```python
from build123d import *

# Parameters (mm, degrees)
SM_BASE_FLANGE_1_OUTLINE_W       = 220
SM_BASE_FLANGE_1_OUTLINE_H       = 2
SM_BASE_FLANGE_1_DEPTH           = 50
HOLE_WIZARD_1_AT_2_COUNT         = 2
HOLE_WIZARD_1_AT_2_PITCH         = 37.643060449
HOLE_WIZARD_1_AT_3_COUNT         = 2
HOLE_WIZARD_1_AT_3_PITCH         = 37.643060449
HOLE_WIZARD_4_2_4_2_1_D          = 4.2
SM_EDGE_FLANGE_1_STRIP_W         = 10
SM_EDGE_FLANGE_1_STRIP_H         = 2
SM_EDGE_FLANGE_1_STRIP_CUT_DEPTH = 220
SM_EDGE_FLANGE_1_DEPTH           = 220
SKETCH_16_W                      = 200
SKETCH_16_H                      = 58
CUT_EXTRUDE_1_DEPTH              = 3
SM_EDGE_FLANGE_2_DEPTH           = 24
HOLE_START                       = 48
HOLE_WIZARD_4_2_4_2_1_2_DEPTH    = 2
FILLET_1_R                       = 5
SKETCH_23_W                      = 1.25
SKETCH_23_H                      = 35
HOLE_WIZARD_M3_1_AT_2_COUNT      = 2
HOLE_WIZARD_M3_1_AT_2_PITCH      = 18.5


# Read off the part's stored shape, not the designer's step: 基体-法兰1, Ø4.2 (4.2) 直径槽口1
# Sheet-metal steps are written as plain solids
with BuildPart() as part:
    # 基体-法兰1 outline → 基体-法兰1 (new body)
    with BuildSketch(Plane.XY):
        with Locations((0, 24)):
            Rectangle(SM_BASE_FLANGE_1_OUTLINE_W, SM_BASE_FLANGE_1_OUTLINE_H)
    extrude(amount=SM_BASE_FLANGE_1_DEPTH)

    # 草图9 → 打孔尺寸(%根据)开槽沉头木螺钉的类型1 (revolve, cut)
    with BuildSketch(Plane(origin=(0, 25, 8.5), x_dir=(0, 0, 1), z_dir=(1, 0, 0))):
        Polygon((0, 0), (0, 2), (1.7, 2), (1.7, 1.6), (3.3, 0), align=None)
    hole_wizard_1 = revolve(axis=Axis((0, 31.35, 8.5), (0, -1, 0)), mode=Mode.SUBTRACT)

    # 打孔尺寸(%根据)开槽沉头木螺钉的类型1 at 2: 打孔尺寸(%根据)开槽沉头木螺钉的类型1 ×2
    with Locations(*[Vector(-0.2922185355990202, 0, 0.956351571051339) * (i * HOLE_WIZARD_1_AT_2_PITCH) for i in range(1, HOLE_WIZARD_1_AT_2_COUNT)]):
        add(hole_wizard_1, mode=Mode.SUBTRACT)

    # 打孔尺寸(%根据)开槽沉头木螺钉的类型1 at 3: 打孔尺寸(%根据)开槽沉头木螺钉的类型1 ×2
    with Locations(*[Vector(0.29221853559902033, 0, 0.956351571051339) * (i * HOLE_WIZARD_1_AT_3_PITCH) for i in range(1, HOLE_WIZARD_1_AT_3_COUNT)]):
        add(hole_wizard_1, mode=Mode.SUBTRACT)

    # Hole Wizard 4.2 _4.2_ _1 (through all)
    with Locations(Plane(origin=(0, 25, 0), x_dir=(1, 0, 0), z_dir=(0, 1, 0))):
        with Locations((-40, -42), (-80, -42), (40, -42), (80, -42)):
            Hole(HOLE_WIZARD_4_2_4_2_1_D / 2)

    # 边线-法兰1 strip (across the edge) → 边线-法兰1 strip cut (cut)
    with BuildSketch(Plane(origin=(110, 23, 50), x_dir=(0, 0, -1), z_dir=(-1, 0, 0))):
        with Locations((-2, -1)):
            Rectangle(SM_EDGE_FLANGE_1_STRIP_W, SM_EDGE_FLANGE_1_STRIP_H)
    extrude(amount=SM_EDGE_FLANGE_1_STRIP_CUT_DEPTH, mode=Mode.SUBTRACT)

    # 边线-法兰1 section (across the edge) → 边线-法兰1 (add)
    with BuildSketch(Plane(origin=(110, 23, 50), x_dir=(0, 0, -1), z_dir=(-1, 0, 0))):
        with BuildLine():
            Line((0, 1), (0, 68))
            Line((0, 68), (2, 68))
            Line((2, 68), (2, 1))
            ThreePointArc((2, 1), (2.292893219, 0.292893219), (3, 0))
            Line((3, 0), (3, -2))
            ThreePointArc((3, -2), (0.878679656, -1.121320344), (0, 1))
        make_face()
    extrude(amount=SM_EDGE_FLANGE_1_DEPTH)

    # 草图16 → 切除-拉伸1 (cut)
    with BuildSketch(Plane.XY.offset(50)):
        with Locations((0, -4)):
            Rectangle(SKETCH_16_W, SKETCH_16_H)
    extrude(amount=-CUT_EXTRUDE_1_DEPTH, mode=Mode.SUBTRACT)

    # 边线-法兰2 section (across the edge) → 边线-法兰2 (add)
    with BuildSketch(Plane(origin=(-12, -10, 48), x_dir=(0, -1, 0), z_dir=(1, 0, 0))):
        with BuildLine():
            Line((0, 1), (0, 35))
            Line((0, 35), (2, 35))
            Line((2, 35), (2, 1))
            ThreePointArc((2, 1), (2.292893219, 0.292893219), (3, 0))
            Line((3, 0), (23, 0))
            Line((23, 0), (23, -2))
            Line((23, -2), (3, -2))
            ThreePointArc((3, -2), (0.878679656, -1.121320344), (0, 1))
        make_face()
    extrude(amount=SM_EDGE_FLANGE_2_DEPTH)

    # Hole Wizard 4.2 _4.2_ _1 2 outline → Hole Wizard 4.2 _4.2_ _1 2 (cut)
    with BuildSketch(Plane.XY.offset(HOLE_START)):
        with BuildLine():
            ThreePointArc((107.1, -2.1), (105, 0), (102.9, -2.1))
            Line((102.9, -2.1), (102.9, -37.9))
            ThreePointArc((102.9, -37.9), (105, -40), (107.1, -37.9))
            Line((107.1, -37.9), (107.1, -2.1))
        make_face()
        with BuildLine():
            Line((-102.9, -37.9), (-102.9, -2.1))
            ThreePointArc((-102.9, -2.1), (-105, 0), (-107.1, -2.1))
            Line((-107.1, -2.1), (-107.1, -37.9))
            ThreePointArc((-107.1, -37.9), (-105, -40), (-102.9, -37.9))
        make_face()
    extrude(amount=HOLE_WIZARD_4_2_4_2_1_2_DEPTH, mode=Mode.SUBTRACT)

    # 圆角1
    fillet_1_edges = [part.edges().sort_by_distance(p)[0] for p in [
        (-110, 24, 0),
        (110, 24, 0),
        (110, -45, 49),
        (-110, -45, 49),
    ]]
    fillet(fillet_1_edges, radius=FILLET_1_R)

    # 草图23 → M3 螺纹孔1 (revolve, cut)
    with BuildSketch(Plane(origin=(9.25, -10, 37), x_dir=(0, 0, 1), z_dir=(1, 0, 0))):
        with Locations((0.625, 17.5)):
            Rectangle(SKETCH_23_W, SKETCH_23_H)
    hole_wizard_m3_1 = revolve(axis=Axis((9.25, -3.65, 37), (0, -1, 0)), mode=Mode.SUBTRACT)

    # M3 螺纹孔1 at 2: M3 螺纹孔1 ×2
    with Locations(*[(-i * HOLE_WIZARD_M3_1_AT_2_PITCH, 0, 0) for i in range(1, HOLE_WIZARD_M3_1_AT_2_COUNT)]):
        add(hole_wizard_m3_1, mode=Mode.SUBTRACT)


solid = part.part
```
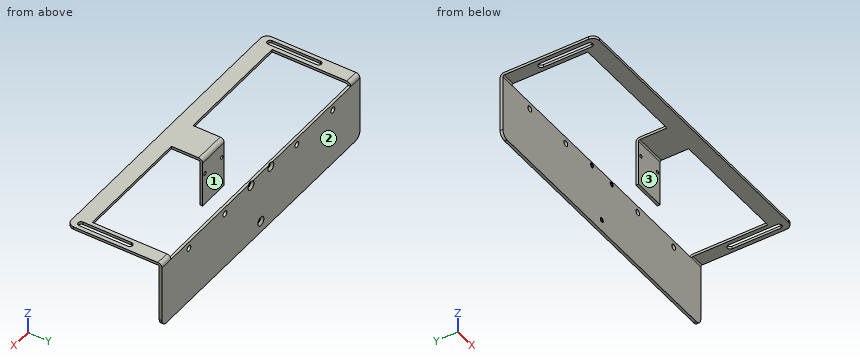
Verification items for the finished model (mm, model axes). Face numbers are marked on the shaded views. A direction names the side the tool comes from. Give positions to 0.01 mm unless a question says otherwise; leave off trailing zeros. Order: outer loops, then holes, each group sorted by start corner. A loop starts at its lowest first (then second) coordinate and runs counter-clockwise, first axis right, second up. Notation, with made-up numbers: M 40.25,51.25 L 64.25,51.25 A26 ccw 64.25,69.25 Z; hole C 30.25,33.25 d6. An arc over 180 degrees is marked long. Answer in a Markdown table with one row per item. Add a question column.
Item 1: Gauge pin test, flat ends, axial feed: pin 1 (3 mm diameter, centred on x = -9.25, z = 37, fed in from -Y); pin 2 (2 mm diameter, centred on x = 0, z = 8.5, fed in from +Y); pin 3 (0.6 mm diameter, centred on x = -1.5, y = -11, fed in from -Z); pin 4 (1.6 mm diameter, centred on x = -53, z = 48.5, fed in from +Y). Record the tip position at first contact, or that the pin passes through.
Item 2: Section check D-D, the plane x = -40. Enter the section's corners in (y, z).
Item 3: Section check B-B, the plane y = -26. Enter the section's corners in (x, z).
Item 4: Tool access check on the marked faces 1, 2 and 3. Record the directions out of +Z, -Z, +X, -X, +Y, -Y that give a thin tool (end or side, any length) a straight path to the whole face; none if there is none.
Item 5: Section check C-C, the plane z = 30.5. Enter the section's corners in (x, y), and give its area (3 significant figures).
Item 6: Section check A-A, the plane x = 90. Enter the section's corners in (y, z).
Item 7: Scan lines: probe 1 along X at (y, z) = (-11.35, 37); probe 2 along X at (y, z) = (23.6, 42); probe 3 along X at (y, z) = (23.3, 44.5). Record each from-to range of solid material in increasing order. Write a range as from..to.
Filled sheet:
| question | item | result |
|---|---|---|
| 1 | pin 1 | stops at y = -12 |
| 1 | pin 2 | passes through |
| 1 | pin 3 | stops at z = 13 |
| 1 | pin 4 | stops at y = -33 |
| 2 | outline | M -45,48 L -33,48 L -33,50 L -45,50 Z; M 23,0 L 25,0 L 25,39.9 L 23,39.9 Z; M 23,44.1 L 25,44.1 L 25,47 L 23,47 Z |
| 3 | outline | M -110,48 L -107.1,48 L -107.1,50 L -110,50 Z; M -102.9,48 L -100,48 L -100,50 L -102.9,50 Z; M -12,48 L 12,48 L 12,50 L -12,50 Z; M 100,48 L 102.9,48 L 102.9,50 L 100,50 Z; M 107.1,48 L 110,48 L 110,50 L 107.1,50 Z |
| 4 | face 1 | +Z, -Z, +X, -X |
| 4 | face 2 | +Z, -Z, +X, -X, +Y |
| 4 | face 3 | -Z, +X, -X, -Y |
| 5 | outline | M -110,23 L 110,23 L 110,25 L -110,25 Z; M -12,-12 L 12,-12 L 12,-10 L -12,-10 Z |
| 5 | area | 488 mm^2 |
| 6 | outline | M -45,48 L -33,48 L -33,50 L -45,50 Z; M 23,0 L 25,0 L 25,47 L 23,47 Z |
| 7 | probe 1 | x = -12..-10.5, -8..8, 10.5..12 |
| 7 | probe 2 | x = -110..-82.1, -77.9..-42.1, -37.9..37.9, 42.1..77.9, 82.1..110 |
| 7 | probe 3 | x = -110..-12.7, -9.3..9.3, 12.7..110 |
